Design review of the part built by this model. Coordinates are the model's own, in mm. Face numbers are marked on the shaded views. Round coordinates to 2 decimals unless told otherwise and drop trailing zeros. Write each loop counter-clockwise with the first axis right and the second up, starting at its lowest first coordinate (ties: lowest second). Pieces come first, ordered by that corner, then holes. Notation, with made-up numbers: (-27, -4.75) -> (12, -4.75) arc R14 ccw to (12, 21.25) -> close; hole circle Ø6 at (80.5, -13.5). An arc over 180 degrees is marked (long way). One line per question, with ' | ' between items. Start each with the question number.
1) Consider section D-D (y = 8). Give the boundary of the cut face in (x, z), then the cut area to 3 significant figures.
2) For probe 1 along X at (y, z) = (7.75, 0); probe 2 along Y at (x, z) = (6, -6), list the stretches that pass through material, from the lowest coordinate up.
3) Consider section C-C (z = 17.5). Give the boundary of the cut face in (x, y) (3 decimals), then the cut area to 3 significant figures.
4) Insertion check: pin 1 Ø1.3 at (x, z) = (1, -21) entering from +Y; pin 2 Ø12 at (x, z) = (-8.5, -6.5) entering from -Y; pin 3 Ø1.5 at (y, z) = (3.5, 2) entering from +X; pin 4 Ø22 at (x, z) = (-2.5, 1.5) entering from +Y. Each pin has a flat end and moves straight along its axis. Give the tip position at first contact, or say it passes through.
5) Consider section A-A (y = 3.75). Give the boundary of the cut face in (x, z) (3 decimals).
6) Mouldability with a two-part tool opening along X and no side actions: class the marked faces 1, 2, 3 and 4 as +X half, -X half, draft (parallel to the pull), parting line (faces both ways), or undercut.
7) Consider section B-B (x = 0). Give the boundary of the cut face in (y, z) (3 decimals).
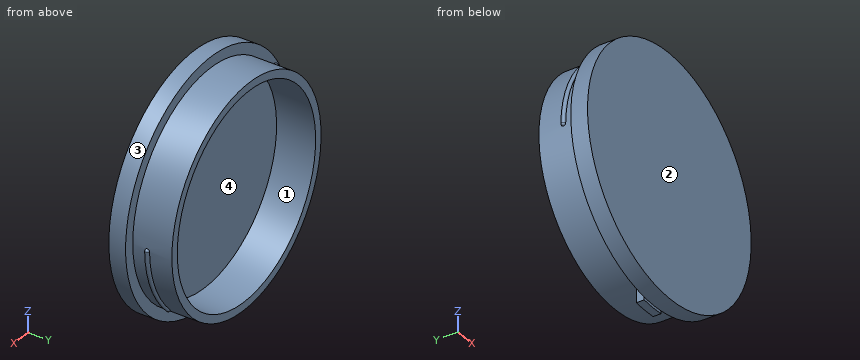
```python
from build123d import *

# Parameters (mm, degrees)
SZKIC1_R                        = 21.875
DODANIE_WYCI_GNI_CIE1_DEPTH     = 3
DODANIE_WYCI_GNI_CIE2_START     = -3
SZKIC2_R                        = 19.95
SZKIC2_R_2                      = 18.5
DODANIE_WYCI_GNI_CIE2_DEPTH     = 10
DODANIE_WYCI_GNI_CIE3_DEPTH     = 1.4
SZKIC4_R                        = 0.4
OBR_T1_ANGLE                    = 45
ZAOKR_GLENIE2_R                 = 0.39
SZYK_KO_OWY5_COUNT              = 2
ZAOKR_GLENIE2_OF_SZYK_KO_OWY5_R = 0.39


with BuildPart() as part:
    # Szkic1 → Dodanie-wyciągnięcie1 (new body)
    with BuildSketch(Plane(origin=(0, 0, 0), x_dir=(1, 0, 0), z_dir=(0, 1, 0))):
        with Locations(Location((0, 0, 0), (0, 0, 270))):
            Circle(SZKIC1_R)
    extrude(amount=DODANIE_WYCI_GNI_CIE1_DEPTH)

    # Szkic2 → Dodanie-wyciągnięcie2 (add)
    with BuildSketch(Plane(origin=(0, 3, 0), x_dir=(1, 0, 0), z_dir=(0, 1, 0)).offset(DODANIE_WYCI_GNI_CIE2_START)):
        with Locations(Location((0, 0, 0), (0, 0, 270))):
            Circle(SZKIC2_R)
        with Locations(Location((0, 0, 0), (0, 0, 270))):
            Circle(SZKIC2_R_2, mode=Mode.SUBTRACT)
    extrude(amount=DODANIE_WYCI_GNI_CIE2_DEPTH)

    # Szkic3 → Dodanie-wyciągnięcie3 (add)
    with BuildSketch(Plane(origin=(0, 3, 0), x_dir=(1, 0, 0), z_dir=(0, 1, 0))):
        with BuildLine():
            Line((-2.25, 22.261584063), (-2.25, 19.822714244))
            ThreePointArc((-2.25, 19.822714244), (0, 19.95), (2.25, 19.822714244))
            Line((2.25, 19.822714244), (2.25, 22.261584063))
            ThreePointArc((2.25, 22.261584063), (0, 22.375), (-2.25, 22.261584063))
        make_face()
    extrude(amount=DODANIE_WYCI_GNI_CIE3_DEPTH)

    # Szkic4 → Obrót1 (revolve)
    with BuildSketch(Plane.XY):
        with Locations((-19.95, 5.6)):
            Circle(SZKIC4_R)
    obr_t1 = revolve(axis=Axis((0, -2.774596357, 0), (0, 1, 0)), revolution_arc=OBR_T1_ANGLE)

    # Zaokrąglenie2
    zaokr_glenie2_edges = [part.edges().sort_by_distance(p)[0] for p in [
        (-14.389622997, 5.6, 14.389622997),
        (-20.35, 5.6, 0),
    ]]
    fillet(zaokr_glenie2_edges, radius=ZAOKR_GLENIE2_R)

    # Szyk kołowy5: Obrót1 ×2 about axis
    szyk_ko_owy5_axis = Axis((0, 10, 0), (0, -1, 0))
    for i in range(1, SZYK_KO_OWY5_COUNT):
        add(obr_t1.rotate(szyk_ko_owy5_axis, i * 360 / SZYK_KO_OWY5_COUNT))

    # Zaokrąglenie2 of Szyk kołowy5
    zaokr_glenie2_of_szyk_ko_owy5_edges = [part.edges().sort_by_distance(p)[0] for p in [
        (14.389622997, 5.6, -14.389622997),
        (20.35, 5.6, 0),
    ]]
    fillet(zaokr_glenie2_of_szyk_ko_owy5_edges, radius=ZAOKR_GLENIE2_OF_SZYK_KO_OWY5_R)


solid = part.part
```
From the geometry:
1) outline: circle Ø39.9 at (0, 0); hole circle Ø37 at (0, 0) | area: 175 mm2
2) probe 1: x = -19.95 to -18.5, 18.5 to 19.95 | probe 2: y = 0 to 3
3) outline: (-13.125, 0) -> (13.125, 0) -> (13.125, 3) -> (9.579, 3) -> (9.579, 10) -> (6, 10) -> (6, 3) -> (-6, 3) -> (-6, 10) -> (-9.579, 10) -> (-9.579, 3) -> (-13.125, 3) -> close | area: 129 mm2
4) pin 1: stops at y = 4.4 | pin 2: stops at y = 0 | pin 3: stops at x = 21.83 | pin 4: stops at y = 3
5) outline: (-2.25, -22.262) arc R22.375 ccw to (2.25, -22.262) -> (2.25, -19.823) arc R19.95 ccw (long way) to (-2.25, -19.823) -> close; hole circle Ø37 at (0, 0)
6) face 1: undercut | face 2: draft | face 3: parting line | face 4: undercut
7) outline: (0, -21.875) -> (3, -21.875) -> (3, -22.375) -> (4.4, -22.375) -> (4.4, -19.95) -> (10, -19.95) -> (10, -18.5) -> (3, -18.5) -> (3, 18.5) -> (10, 18.5) -> (10, 19.95) -> (3, 19.95) -> (3, 21.875) -> (0, 21.875) -> close
